Here's how the part is built. I have some questions about the finished solid (model axes, mm). Round coordinates to 2 decimals unless told otherwise and drop trailing zeros. Loops run counter-clockwise (first coordinate to the right, second up) from the corner with the lowest first, then second, coordinate; pieces in that order, holes last. Notation, with made-up numbers: M 45,74 L 68,74 A22 cw 68,87 Z; hole C -37,71 d9. An arc over 180 degrees is marked long. Use a Markdown table: item, result.
from build123d import *

# Parameters (mm, degrees)
SKETCH1_R                       = 12.7
SKETCH1_R_2                     = 7.14375
BOSS_EXTRUDE1_DEPTH             = 11.1125
FILLET1_R                       = 0.254
F_1_4_0_25_DIAMETER_HOLE1_D     = 6.35
F_1_4_0_25_DIAMETER_HOLE1_DEPTH = 10.922
F_1_4_0_25_DIAMETER_HOLE1_TIP   = 1.907732465


with BuildPart() as part:
    # Sketch1 → Boss-Extrude1 (new body)
    with BuildSketch(Plane.XY):
        Circle(SKETCH1_R)
        Circle(SKETCH1_R_2, mode=Mode.SUBTRACT)
    extrude(amount=BOSS_EXTRUDE1_DEPTH)

    # Fillet1
    fillet1_edges = [part.edges().sort_by_distance(p)[0] for p in [
        (-12.7, 0, 0),
        (-12.7, 0, 11.1125),
        (-7.14375, 0, 0),
        (-7.14375, 0, 11.1125),
    ]]
    fillet(fillet1_edges, radius=FILLET1_R)

    # 1/4 (0.25) Diameter Hole1
    with Locations(Plane(origin=(-0.017095138, 12.699988494, 5.351108343), x_dir=(0.999999094, 0.001346074, 0), z_dir=(-0.001346074, 0.999999094, 0))):
        with Locations((0, 0)):
            Hole(F_1_4_0_25_DIAMETER_HOLE1_D / 2, depth=F_1_4_0_25_DIAMETER_HOLE1_DEPTH)
            with Locations((0, 0, -(F_1_4_0_25_DIAMETER_HOLE1_DEPTH + F_1_4_0_25_DIAMETER_HOLE1_TIP / 2))):  # 118° drill point
                Cone(0, F_1_4_0_25_DIAMETER_HOLE1_D / 2, F_1_4_0_25_DIAMETER_HOLE1_TIP, mode=Mode.SUBTRACT)


solid = part.part
1. For pin 1 Ø5 at (x, z) = (3, 6) entering from +Y; pin 2 Ø8.5 at (x, y) = (0, 0) entering from -Z; pin 3 Ø6 at (x, z) = (8, 4) entering from +Y, each with a flat end and sliding along its axis, tell me the tip position at first contact or that it passes through.
Answer sheet:
| item | result |
|---|---|
| pin 1 | y = 12.6 |
| pin 2 | through |
| pin 3 | y = 11.67 |
2. Imagine slicing it at C-C, the plane z = 4.25. Write out the boundary of the cut face in (x, y), then the cut area to 3 significant figures.
Answer sheet:
| item | result |
|---|---|
| outline | M -2.99,6.49 L -2.99,12.34 A12.7 ccw long 2.96,12.35 L 2.97,6.5 A7.14 cw long Z |
| area | 313 mm2 |
3. We'd pull the mould along Y, two halves only. Please class faces 1 (the face through (-2.75, -12.4, 5.48)), 2 (the face through (5.4, -5.4, 11.112)), 3 (the face through (-1.549, -6.974, 5.482)): +Y half, -Y half, draft (parallel to the pull), parting line (faces both ways), or undercut.
Answer sheet:
| item | result |
|---|---|
| face 1 | parting line |
| face 2 | draft |
| face 3 | undercut |
4. Imagine slicing it at D-D, the plane z = 7.5. Write out the boundary of the cut face in (x, y).
Answer sheet:
| item | result |
|---|---|
| outline | M -2.35,6.75 L -2.35,12.48 A12.7 ccw long 2.32,12.49 L 2.33,6.75 A7.14 cw long Z |
5. I need wall thicknesses on probe 1 along X at (y, z) = (0.25, 9.5); probe 2 along Y at (x, z) = (-3, 4); probe 3 along Y at (x, z) = (0, 7.75). Which ranges of each line are inside material? Lowest first, please. Write a range as from..to.
Answer sheet:
| item | result |
|---|---|
| probe 1 | -12.7..-7.14, 7.14..12.7 |
| probe 2 | -12.34..-6.48, 6.48..12.34 |
| probe 3 | -12.7..-7.14 |
6. Imagine slicing it at B-B, the plane x = 0. State how many separate pieces and enclosed holes the cut face has, then the cut area to 3 significant figures.
Answer sheet:
| item | result |
|---|---|
| separate pieces | 3 |
| enclosed holes | 0 |
| area | 88.1 mm2 |
7. Imagine slicing it at A-A, the plane y = 0. Write out the boundary of the cut face in (x, z), then the cut area to 3 significant figures.
Answer sheet:
| item | result |
|---|---|
| outline | M -12.7,0.25 A0.25 ccw -12.45,0 L -7.4,0 A0.25 ccw -7.14,0.25 L -7.14,10.86 A0.25 ccw -7.4,11.11 L -12.45,11.11 A0.25 ccw -12.7,10.86 Z; M 7.14,0.25 A0.25 ccw 7.4,0 L 12.45,0 A0.25 ccw 12.7,0.25 L 12.7,10.86 A0.25 ccw 12.45,11.11 L 7.4,11.11 A0.25 ccw 7.14,10.86 Z |
| area | 123 mm2 |
